Geometry: final body of the model. Coordinates: model frame, mm. A direction names the side the tool comes from. Give positions to 0.01 mm unless a question says otherwise; leave off trailing zeros. Loops run counter-clockwise (first coordinate to the right, second up) from the corner with the lowest first, then second, coordinate; pieces in that order, holes last. Notation, with made-up numbers: M 74,81 L 100,81 A24 cw 100,102 Z; hole C -22.5,57.25 d1. An arc over 180 degrees is marked long. Put each result on its own line as item: value.
Autodesk Fusion 360 part; units mm, degrees
sketch "Skizze1" plane through (0, 0, 0) normal (0, 1, 0) x (1, 0, 0)
  line L0 (-28.3, 2.34) -> (28.3, 2.34)
  line L1 (28.3, -26.86) -> (-28.3, -26.86)
  line L2 (0, -1.75) -> (0, -22.5)
  circle A0 centre (28.3, -22.03) radius 1.1
  circle A1 centre (-28.3, -22.03) radius 1.1
  line L3 (-22.6, 2.09) -> (27.9, 2.09)
  line L4 (27.9, 2.09) -> (27.9, -17.21)
  line L5 (27.9, -17.21) -> (-22.6, -17.21)
  line L6 (-22.6, -17.21) -> (-22.6, 2.09)
  line L7 (-28.3, -20.23) -> (-28.3, 2.34)
  line L8 (28.3, 2.34) -> (28.3, -20.23)
  line L9 (28.3, -23.83) -> (28.3, -26.86)
  arc A2 (28.3, -23.83) -> (28.3, -20.23) centre (28.3, -22.03) ccw
  arc A3 (-28.3, -20.23) -> (-28.3, -23.83) centre (-28.3, -22.03) ccw
  line L10 (-28.3, -26.86) -> (-28.3, -23.83)
  line L11 (-19.3, -27.66) -> (-26.3, -27.66)
  line L12 (-26.3, -27.66) -> (-26.3, -20.46)
  line L13 (-26.3, -20.46) -> (-19.3, -20.46)
  line L14 (-19.3, -20.46) -> (-19.3, -27.66)
  line L15 (15.05, -19.75) -> (20.9, -19.75)
  line L16 (20.9, -19.75) -> (20.9, -27.62)
  line L17 (20.9, -27.62) -> (15.05, -27.62)
  line L18 (15.05, -27.62) -> (15.05, -19.75)
  dimension "d3" = 29.2
  dimension "d4" = 56.6
  dimension "d5" = 4.83
  dimension "d6" = 3.6
  dimension "d7" = 2.2
  dimension "d8" = 5.7
  dimension "d9" = 50.5
  dimension "d10" = 19.3
  dimension "d11" = 0.25
  dimension "d17" = 2
  dimension "d19" = 0.8
  dimension "d20" = 6.4
  dimension "d21" = 7
  dimension "d22" = 7.4
  dimension "d23" = 5.85
  dimension "d24" = 0.76
  dimension "d25" = 7.11
extrude "Extrusion1" add sketch "Skizze1" along normal blind 1.6 contours L0 L1 L7 L8 L9 A2 A3 L10 L12 L13 L14 L15 L16 L18 | L1 L12 L13 L14 | L1 L15 L16 L18 | L3 L4 L5 L6
extrude "Extrusion2" add sketch "Skizze1" along normal blind 8.2 from surface at 1.6 contours L3 L4 L5 L6
extrude "Extrusion3" add sketch "Skizze1" along normal blind 4 from surface at 1.6 contours L1 L12 L13 L14 | L1 L11 L12 L14 | L1 L16 L17 L18 | L1 L15 L16 L18
Item 1: Section A-A on z = 22.03. Output: boundary loops of the cut face in (x, y).
Output values:
outline: M -30.1,0 L -29.4,0 L -29.4,1.6 L -30.1,1.6 Z; M -27.2,0 L 27.2,0 L 27.2,1.6 L 20.9,1.6 L 20.9,5.6 L 15.05,5.6 L 15.05,1.6 L -19.3,1.6 L -19.3,5.6 L -26.3,5.6 L -26.3,1.6 L -27.2,1.6 Z; M 29.4,0 L 30.1,0 L 30.1,1.6 L 29.4,1.6 Z
Item 2: Pin query (flat end, axial travel): pin 1 Ø0.5 at (y, z) = (1, 25.5) entering from +X; pin 2 Ø3 at (y, z) = (4.5, 23.5) entering from +X; pin 3 Ø0.8 at (y, z) = (1, 14) entering from -X. Return the tip coordinate at first contact, or that it passes through.
Output values:
pin 1: x = 28.3
pin 2: x = 20.9
pin 3: x = -28.3
Item 3: Mould query, pull axis X, two halves, no side actions, for faces 1 (the flat face through (3, 6, 17.21)), 2 (the cylindrical face through (-28.44, 0.79, 23.12)), 3 (the flat face through (20.9, 4, 24)), 4 (the flat face through (15.05, 4, 24)). Classes: pulls with the +X half, pulls with the -X half, needs draft (parallel to the pull), parting line crosses it, or undercut.
Output values:
face 1: needs draft
face 2: undercut
face 3: pulls with the +X half
face 4: undercut
Item 4: Section D-D on z = 2.25. Output: boundary loops of the cut face in (x, y).
Output values:
outline: M -28.3,0 L 28.3,0 L 28.3,1.6 L 27.9,1.6 L 27.9,9.8 L -22.6,9.8 L -22.6,1.6 L -28.3,1.6 Z
Item 5: Section B-B on y = 2.75. Output: boundary loops of the cut face in (x, z).
Output values:
outline: M -26.3,20.46 L -19.3,20.46 L -19.3,27.66 L -26.3,27.66 Z; M -22.6,-2.09 L 27.9,-2.09 L 27.9,17.21 L -22.6,17.21 Z; M 15.05,19.75 L 20.9,19.75 L 20.9,27.62 L 15.05,27.62 Z
Item 6: Section C-C on x = -8. Output: boundary loops of the cut face in (y, z).
Output values:
outline: M 0,-2.34 L 1.6,-2.34 L 1.6,-2.09 L 9.8,-2.09 L 9.8,17.21 L 1.6,17.21 L 1.6,26.86 L 0,26.86 Z
Item 7: Set-up query: faces 5 (the flat face through (-28.3, 1, 25)), 6 (the flat face through (0, 1, 26.86)), 7 (the flat face through (2, 6, -2.09)), 8 (the flat face through (-28.3, 1, 9)). Return all of +Z, -Z, +X, -X, +Y, -Y with unobstructed straight access to the full face (end or side cutting, diameter ignored); none if empty.
Output values:
face 5: +Z, -X, +Y, -Y
face 6: +Z, +X, -X, -Y
face 7: -Z, +X, -X, +Y
face 8: -Z, -X, +Y, -Y
Item 8: Line query: probe 1 along X at (y, z) = (1, 22.03); probe 2 along Z at (x, y) = (19, 4.25); probe 3 along X at (y, z) = (3.25, 25.5). Output: solid intervals per line, ascending. Write a range as [from, to].
Output values:
probe 1: [-30.1, -29.4], [-27.2, 27.2], [29.4, 30.1]
probe 2: [-2.09, 17.21], [19.75, 27.62]
probe 3: [-26.3, -19.3], [15.05, 20.9]
